Read the model definition and answer for the solid it produces. Units are mm, in the model's axes. A direction names the side the tool comes from. Coordinates: 2 decimals unless noted, no trailing zeros. Loops run counter-clockwise (first coordinate to the right, second up) from the corner with the lowest first, then second, coordinate; pieces in that order, holes last. Notation, with made-up numbers: M -33,29 L -28,29 A20 ccw -28,51 Z; hole C -3.75,5.25 d3. An arc over 180 degrees is marked long. Use one line per item in the form item = value. Start each with the question number.
1. For a pull along X with two mould halves and no side action, classify faces 4 (the flat face through (0, -1.085, 2)), 5 (the cylindrical face through (-0.05, 1.7, 1.98)), 6 (the cylindrical face through (2.146, 0.676, 2.232)), 7 (the flat face through (0, -2, 0.5)) as released by +X, released by -X, zero draft, split by the parting line, or undercut.
2. Find the intervals of material crossed by probe 1 along Y at (x, z) = (0, 1.95); probe 2 along Z at (x, y) = (-1.95, 0); probe 3 along X at (y, z) = (0, 1.6), in increasing order. Write a range as [from, to].
3. The part is cut by section C-C (z = 3). Give the vertices of the cut face in (x, y).
4. A flat-ended cylindrical pin translates along its axis: pin 1 (1.3 mm diameter, centred on x = 0, z = 2, fed in from +Y). Find the tip coordinate at first contact, or state that the pin passes through.
5. The part is cut by section A-A (x = 0). Give the vertices of the cut face in (y, z), plus the area to 3 significant figures.
6. The part is cut by section D-D (z = 2.1). Give the vertices of the cut face in (x, y).
7. A tool of negligible diameter and unlimited length cuts with its end or side. For faces 1 (the flat face through (2, -2, 1)), 2 (the cylindrical face through (-1.9, -0.3, 2.4)), 3 (the cylindrical face through (0.802, 3.612, 0.746)), from which of +Z, -Z, +X, -X, +Y, -Y can it reach the whole face along a straight path? Write none if from no direction.
8. The part is cut by section B-B (y = 0). Give the vertices of the cut face in (x, z).
from build123d import *
from build123d.topology import SkipClean

# Parameters (mm, degrees)
ESBO_O1_R                    = 3.7
RESSALTO_EXTRUS_O2_DEPTH     = 6.5
ESBO_O2_R                    = 1.875
CORTE_EXTRUS_O1_DEPTH        = 0.6
ESBO_O3_R                    = 5
ESBO_O3_R_2                  = 2.415
CORTE_EXTRUS_O2_DEPTH        = 5.5
ESBO_O6_R                    = 2.05
CORTE_EXTRUS_O6_DEPTH        = 0.9
ESBO_O7_R                    = 2.415
ESBO_O7_R_2                  = 2.1
CORTE_EXTRUS_O7_DEPTH        = 5.5
RESSALTO_EXTRUS_O3_START     = 3.5
ESBO_O8_R                    = 2.25
ESBO_O8_R_2                  = 2.1
RESSALTO_EXTRUS_O3_DEPTH     = 3.5
RESSALTO_EXTRUS_O4_START     = 3.5
ESBO_O11_R                   = 2.65
ESBO_O11_R_2                 = 2.25
RESSALTO_EXTRUS_O4_DEPTH     = 3.5
ESBO_O9_R                    = 0.5
CORTE_EXTRUS_O8_DEPTH        = 10
ESBO_O13_R                   = 3.7
CORTE_EXTRUS_O10_DEPTH       = 0.5
ESBO_O14_R                   = 2.05
CORTE_EXTRUS_O11_DEPTH       = 0.4
ESBO_O15_W                   = 5.3
ESBO_O15_H                   = 2.277962938
CORTE_EXTRUS_O12_DEPTH       = 5.2
RESSALTO_EXTRUS_O6_START     = 0.8
ESBO_O17_R                   = 2.05
RESSALTO_EXTRUS_O6_DEPTH     = 0.8
CORTE_EXTRUS_O13_START       = -3.5
CORTE_EXTRUS_O13_OUTLINE_R   = 2.65
CORTE_EXTRUS_O13_OUTLINE_R_2 = 2.25
CORTE_EXTRUS_O13_DEPTH       = 3.5
ESBO_O19_W                   = 1.26014474
ESBO_O19_H                   = 6.353969252
CORTE_EXTRUS_O14_DEPTH       = 5
CORTE_EXTRUS_O15_DEPTH       = 10


# Read off the part's stored shape, not the designer's step: Corte-extrusão13
with BuildPart() as part:
    # Esboço1 → Ressalto-extrusão2 (new body)
    with BuildSketch(Plane.XY):
        with Locations(Location((0, 0, 0), (0, 0, 180))):
            Circle(ESBO_O1_R)
        with BuildLine():
            Line((-1.211385827, -0.884615385), (1.211385827, -0.884615385))
            ThreePointArc((1.211385827, -0.884615385), (0, 1.5), (-1.211385827, -0.884615385))
        make_face(mode=Mode.SUBTRACT)
    extrude(amount=RESSALTO_EXTRUS_O2_DEPTH)

    # Esboço2 → Corte-extrusão1 (cut)
    with BuildSketch(Plane(origin=(0, 0, 0), x_dir=(-1, 0, 0), z_dir=(0, 0, -1))):
        Circle(ESBO_O2_R)
    extrude(amount=-CORTE_EXTRUS_O1_DEPTH, mode=Mode.SUBTRACT)

    # Esboço3 → Corte-extrusão2 (cut)
    with BuildSketch(Plane.XY.offset(6.5)):
        Circle(ESBO_O3_R)
        Circle(ESBO_O3_R_2, mode=Mode.SUBTRACT)
    extrude(amount=-CORTE_EXTRUS_O2_DEPTH, mode=Mode.SUBTRACT)

    # Esboço6 → Corte-extrusão6 (cut)
    with BuildSketch(Plane(origin=(0, 0, 0), x_dir=(-1, 0, 0), z_dir=(0, 0, -1))):
        Circle(ESBO_O6_R)
    extrude(amount=-CORTE_EXTRUS_O6_DEPTH, mode=Mode.SUBTRACT)

    # Esboço7 → Corte-extrusão7 (cut)
    with BuildSketch(Plane.XY.offset(6.5)):
        Circle(ESBO_O7_R)
        Circle(ESBO_O7_R_2, mode=Mode.SUBTRACT)
    extrude(amount=-CORTE_EXTRUS_O7_DEPTH, mode=Mode.SUBTRACT)

    # Esboço8 → Ressalto-extrusão3 (add)
    with BuildSketch(Plane.XY.offset(1).offset(RESSALTO_EXTRUS_O3_START)):
        Circle(ESBO_O8_R)
        Circle(ESBO_O8_R_2, mode=Mode.SUBTRACT)
    extrude(amount=-RESSALTO_EXTRUS_O3_DEPTH)

    # Esboço11 → Ressalto-extrusão4 (add)
    with BuildSketch(Plane.XY.offset(1).offset(RESSALTO_EXTRUS_O4_START)):
        Circle(ESBO_O11_R)
        Circle(ESBO_O11_R_2, mode=Mode.SUBTRACT)
    extrude(amount=-RESSALTO_EXTRUS_O4_DEPTH)

    # Esboço9 → Corte-extrusão8 (cut)
    with BuildSketch(Plane(origin=(0, 0, 0), x_dir=(0, 0, -1), z_dir=(1, 0, 0))):
        with Locations((-2, 0)):
            Circle(ESBO_O9_R)
    extrude(amount=-CORTE_EXTRUS_O8_DEPTH, mode=Mode.SUBTRACT)

    # Esboço13 → Corte-extrusão10 (cut)
    with BuildSketch(Plane(origin=(0, 0, 0), x_dir=(-1, 0, 0), z_dir=(0, 0, -1))):
        Circle(ESBO_O13_R)
    extrude(amount=-CORTE_EXTRUS_O10_DEPTH, mode=Mode.SUBTRACT)

    # Esboço14 → Corte-extrusão11 (cut)
    with BuildSketch(Plane(origin=(0, 0, 0.9), x_dir=(-1, 0, 0), z_dir=(0, 0, -1))):
        Circle(ESBO_O14_R)
    extrude(amount=-CORTE_EXTRUS_O11_DEPTH, mode=Mode.SUBTRACT)

    # Esboço15 → Corte-extrusão12 (cut, symmetric)
    with BuildSketch(Plane(origin=(0, 0, 0), x_dir=(1, 0, 0), z_dir=(0, 1, 0))):
        with Locations((0, -5.638981469)):
            Rectangle(ESBO_O15_W, ESBO_O15_H)
    extrude(amount=CORTE_EXTRUS_O12_DEPTH, both=True, mode=Mode.SUBTRACT)

    # Esboço17 → Ressalto-extrusão6 (add)
    with SkipClean():  # the faces are left unmerged after this step: merging them gives an invalid solid
        with BuildSketch(Plane(origin=(0, 0, 1.3), x_dir=(-1, 0, 0), z_dir=(0, 0, -1)).offset(RESSALTO_EXTRUS_O6_START)):
            Circle(ESBO_O17_R)
            with BuildLine():
                Line((-1.211385827, -0.884615385), (1.211385827, -0.884615385))
                ThreePointArc((1.211385827, -0.884615385), (0, 1.5), (-1.211385827, -0.884615385))
            make_face(mode=Mode.SUBTRACT)
        extrude(amount=-RESSALTO_EXTRUS_O6_DEPTH)

    # Corte-extrusão13 outline → Corte-extrusão13 (cut)
    with SkipClean():  # the faces are left unmerged after this step: merging them gives an invalid solid
        with BuildSketch(Plane.XY.offset(4.5).offset(CORTE_EXTRUS_O13_START)):
            Circle(CORTE_EXTRUS_O13_OUTLINE_R)
            Circle(CORTE_EXTRUS_O13_OUTLINE_R_2, mode=Mode.SUBTRACT)
        extrude(amount=CORTE_EXTRUS_O13_DEPTH, mode=Mode.SUBTRACT)

    # Esboço19 → Corte-extrusão14 (cut, symmetric)
    with SkipClean():  # the faces are left unmerged after this step: merging them gives an invalid solid
        with BuildSketch(Plane(origin=(0, 0, 0), x_dir=(0, 0, -1), z_dir=(1, 0, 0))):
            with Locations((-4.13007237, -0.123588244)):
                Rectangle(ESBO_O19_W, ESBO_O19_H)
        extrude(amount=CORTE_EXTRUS_O14_DEPTH, both=True, mode=Mode.SUBTRACT)

    # Esboço20 → Corte-extrusão15 (cut)
    with BuildSketch(Plane(origin=(0, 0, 0.5), x_dir=(-1, 0, 0), z_dir=(0, 0, -1))):
        with BuildLine():
            Line((-1.30904907, -1.084615385), (1.30904907, -1.084615385))
            ThreePointArc((1.30904907, -1.084615385), (0, 1.7), (-1.30904907, -1.084615385))
        make_face()
    extrude(amount=-CORTE_EXTRUS_O15_DEPTH, mode=Mode.SUBTRACT)


solid = part.part
Computed values:
q1.face_4 = undercut
q1.face_5 = undercut
q1.face_6 = split by the parting line
q1.face_7 = zero draft
q2.probe_1 = [-2.25, -1.08], [1.7, 2.25]
q2.probe_2 = [0.5, 1.5], [2.5, 3.5]
q2.probe_3 = [1.7, 2.25]
q3.outline = C 0,0 d4.5; hole M -1.31,-1.08 L 1.31,-1.08 A1.7 ccw long Z
q4.pin_1 = 2.25
q5.outline = M -3.7,0.5 L -1.08,0.5 L -1.08,3.5 L -2.25,3.5 L -2.25,1 L -3.7,1 Z; M 1.7,0.5 L 3.7,0.5 L 3.7,1 L 2.25,1 L 2.25,3.5 L 1.7,3.5 Z
q5.area = 6.60 mm²
q6.outline = M -2.2,-0.49 A2.25 ccw long -2.2,0.49 L -1.63,0.49 A1.7 cw long 1.31,-1.08 L -1.31,-1.08 A1.7 cw -1.63,-0.49 Z
q7.face_1 = +Z
q7.face_2 = -X
q7.face_3 = +Z, -Z
q8.outline = M -3.7,0.5 L -1.7,0.5 L -1.7,1.5 L -2.25,1.5 L -2.25,1 L -3.7,1 Z; M -2.25,2.5 L -1.7,2.5 L -1.7,3.5 L -2.25,3.5 Z; M 1.7,0.5 L 3.7,0.5 L 3.7,1 L 2.25,1 L 2.25,3.5 L 1.7,3.5 Z
